Model file for the job. Use its own axes, mm. Give positions to 0.01 mm unless a question says otherwise; leave off trailing zeros. Write each loop counter-clockwise with the first axis right and the second up, starting at its lowest first coordinate (ties: lowest second). Pieces come first, ordered by that corner, then holes. Notation, with made-up numbers: (4.5, 45) - (63.5, 45) arc R16 ccw to (63.5, 54) - close; hole circle Ø10 at (-10, 18). An arc over 180 degrees is marked (long way). One line per item, written item: value. Start each with the question number.
(1) Cut at C-C, the plane y = 1.6. List the corners of the cut face in (x, z) (3 decimals), and give its area (3 significant figures).
(2) Probe L1, parallel to X at y = 0.8, z = -1; L2, parallel to X at y = 0.5, z = 32; L3, parallel to Z at x = -14.5, y = 1.05. List the from-to ranges inside material, lowest first.
(3) Cut at B-B, the plane z = 0. List the corners of the cut face in (x, y), and give its area (3 significant figures).
(4) Cut at A-A, the plane x = 0. List the corners of the cut face in (y, z), and give its area (3 significant figures).
(5) Cut at D-D, the plane x = -18. List the corners of the cut face in (y, z).
(6) Drop flat-ended pins along their axis: P1, Ø1.5, axis at y = 2, z = -6.5, coming from the -X side; P2, Ø1.8, axis at x = 28.8, z = 16.63, coming from the +Y side; P3, Ø1, axis at x = -25, y = 2.5, coming from the -Z side; P4, Ø1.5, axis at y = 0.5, z = 7, coming from the +X side. Give the stop position or say it passes through.
(7) Mould opens along Z. For faces 1 (the face through (-30.283, 1.521, -16.43)), 2 (the face through (-29.4, 3, 7.9)), 3 (the face through (10.889, 1.479, 34.576)) say: pulls with the +Z half, pulls with the -Z half, needs draft (parallel to the pull), parting line crosses it, or undercut.
from build123d import *

# Parameters (mm, degrees)
SKETCH1_R           = 36.25
SKETCH1_R_2         = 30.25
BOSS_EXTRUDE1_DEPTH = 3
SKETCH2_R           = 1.5
CUT_EXTRUDE1_DEPTH  = 52.352945388
CIRPATTERN1_COUNT   = 6


with BuildPart() as part:
    # Sketch1 → Boss-Extrude1 (new body)
    with BuildSketch(Plane(origin=(0, 0, 0), x_dir=(1, 0, 0), z_dir=(0, 1, 0))):
        with Locations(Location((0, 0, 0), (0, 0, 270))):
            Circle(SKETCH1_R)
        with Locations(Location((0, 0, 0), (0, 0, 270))):
            Circle(SKETCH1_R_2, mode=Mode.SUBTRACT)
    extrude(amount=BOSS_EXTRUDE1_DEPTH)

    # Sketch2 → Cut-Extrude1 (cut, symmetric)
    with BuildSketch(Plane(origin=(0, 3, 0), x_dir=(1, 0, 0), z_dir=(0, 1, 0))):
        with Locations(Location((0, 33.25, 0), (0, 0, 270))):
            Circle(SKETCH2_R)
    cut_extrude1 = extrude(amount=CUT_EXTRUDE1_DEPTH, both=True, mode=Mode.SUBTRACT)

    # CirPattern1: Cut-Extrude1 ×6 about axis
    cirpattern1_axis = Axis((0, 0, 0), (0, 1, 0))
    for i in range(1, CIRPATTERN1_COUNT):
        add(cut_extrude1.rotate(cirpattern1_axis, i * 360 / CIRPATTERN1_COUNT), mode=Mode.SUBTRACT)


solid = part.part
Answers follow:
1. outline: circle Ø72.5 at (0, 0); hole circle Ø3 at (-28.795, -16.625); hole circle Ø3 at (-28.795, 16.625); hole circle Ø60.5 at (0, 0); hole circle Ø3 at (0, -33.25); hole circle Ø3 at (0, 33.25); hole circle Ø3 at (28.795, -16.625); hole circle Ø3 at (28.795, 16.625)
1. area: 1,210 mm²
2. L1: x = -36.24 to -30.23, 30.23 to 36.24
2. L2: x = -17.03 to -0.83, 0.83 to 17.03
2. L3: z = -33.22 to -26.55, 26.55 to 33.22
3. outline: (-36.25, 0) - (-30.25, 0) - (-30.25, 3) - (-36.25, 3) - close; (30.25, 0) - (36.25, 0) - (36.25, 3) - (30.25, 3) - close
3. area: 36.0 mm²
4. outline: (0, -36.25) - (3, -36.25) - (3, -34.75) - (0, -34.75) - close; (0, -31.75) - (3, -31.75) - (3, -30.25) - (0, -30.25) - close; (0, 30.25) - (3, 30.25) - (3, 31.75) - (0, 31.75) - close; (0, 34.75) - (3, 34.75) - (3, 36.25) - (0, 36.25) - close
4. area: 18.0 mm²
5. outline: (0, -31.47) - (3, -31.47) - (3, -24.31) - (0, -24.31) - close; (0, 24.31) - (3, 24.31) - (3, 31.47) - (0, 31.47) - close
6. P1: stops at x = -35.79
6. P2: passes through
6. P3: stops at z = -26.72
6. P4: stops at x = 35.71
7. face 1: undercut
7. face 2: needs draft
7. face 3: parting line crosses it
